from build123d import *

# Parameters (mm, degrees)
SKETCH2_R           = 1
BOSS_EXTRUDE1_DEPTH = 110


with BuildPart() as part:
    # Sketch2 → Boss-Extrude1 (new body)
    with BuildSketch(Plane.XY):
        with BuildLine():
            Line((0, 2.5), (1.335786438, 2.5))
            ThreePointArc((1.335786438, 2.5), (1.431457296, 2.519030117), (1.512563133, 2.573223305))
            Line((1.512563133, 2.573223305), (3.012563133, 4.073223305))
            ThreePointArc((3.012563133, 4.073223305), (3.066756321, 4.345670858), (2.835786438, 4.5))
            Line((2.835786438, 4.5), (1.25, 4.5))
            ThreePointArc((1.25, 4.5), (1.073223305, 4.573223305), (1, 4.75))
            Line((1, 4.75), (1, 5.75))
            ThreePointArc((1, 5.75), (1.073223305, 5.926776695), (1.25, 6))
            Line((1.25, 6), (5.75, 6))
            ThreePointArc((5.75, 6), (5.926776695, 5.926776695), (6, 5.75))
            Line((6, 5.75), (6, 1.25))
            ThreePointArc((6, 1.25), (5.926776695, 1.073223305), (5.75, 1))
            Line((5.75, 1), (4.748585621, 1))
            ThreePointArc((4.748585621, 1), (4.571808926, 1.073223305), (4.498585621, 1.25))
            Line((4.498585621, 1.25), (4.498585621, 2.834372059))
            ThreePointArc((4.498585621, 2.834372059), (4.344256479, 3.065341942), (4.071808926, 3.011148754))
            Line((4.071808926, 3.011148754), (2.573223305, 1.512563133))
            ThreePointArc((2.573223305, 1.512563133), (2.519030117, 1.431457296), (2.5, 1.335786438))
            Line((2.5, 1.335786438), (2.5, -1.335786438))
            ThreePointArc((2.5, -1.335786438), (2.519030117, -1.431457296), (2.573223305, -1.512563133))
            Line((2.573223305, -1.512563133), (4.071808926, -3.011148754))
            ThreePointArc((4.071808926, -3.011148754), (4.344256479, -3.065341942), (4.498585621, -2.834372059))
            Line((4.498585621, -2.834372059), (4.498585621, -1.25))
            ThreePointArc((4.498585621, -1.25), (4.571808926, -1.073223305), (4.748585621, -1))
            Line((4.748585621, -1), (5.75, -1))
            ThreePointArc((5.75, -1), (5.926776695, -1.073223305), (6, -1.25))
            Line((6, -1.25), (6, -5.75))
            ThreePointArc((6, -5.75), (5.926776695, -5.926776695), (5.75, -6))
            Line((5.75, -6), (1.25, -6))
            ThreePointArc((1.25, -6), (1.073223305, -5.926776695), (1, -5.75))
            Line((1, -5.75), (1, -4.75))
            ThreePointArc((1, -4.75), (1.073223305, -4.573223305), (1.25, -4.5))
            Line((1.25, -4.5), (2.835786438, -4.5))
            ThreePointArc((2.835786438, -4.5), (3.066756321, -4.345670858), (3.012563133, -4.073223305))
            Line((3.012563133, -4.073223305), (1.512563133, -2.573223305))
            ThreePointArc((1.512563133, -2.573223305), (1.431457296, -2.519030117), (1.335786438, -2.5))
            Line((1.335786438, -2.5), (-1.335786438, -2.5))
            ThreePointArc((-1.335786438, -2.5), (-1.431457296, -2.519030117), (-1.512563133, -2.573223305))
            Line((-1.512563133, -2.573223305), (-3.012563133, -4.073223305))
            ThreePointArc((-3.012563133, -4.073223305), (-3.066756321, -4.345670858), (-2.835786438, -4.5))
            Line((-2.835786438, -4.5), (-1.25, -4.5))
            ThreePointArc((-1.25, -4.5), (-1.073223305, -4.573223305), (-1, -4.75))
            Line((-1, -4.75), (-1, -5.75))
            ThreePointArc((-1, -5.75), (-1.073223305, -5.926776695), (-1.25, -6))
            Line((-1.25, -6), (-5.75, -6))
            ThreePointArc((-5.75, -6), (-5.926776695, -5.926776695), (-6, -5.75))
            Line((-6, -5.75), (-6, -1.25))
            ThreePointArc((-6, -1.25), (-5.926776695, -1.073223305), (-5.75, -1))
            Line((-5.75, -1), (-4.748585621, -1))
            ThreePointArc((-4.748585621, -1), (-4.571808926, -1.073223305), (-4.498585621, -1.25))
            Line((-4.498585621, -1.25), (-4.498585621, -2.834372059))
            ThreePointArc((-4.498585621, -2.834372059), (-4.344256479, -3.065341942), (-4.071808926, -3.011148754))
            Line((-4.071808926, -3.011148754), (-2.573223305, -1.512563133))
            ThreePointArc((-2.573223305, -1.512563133), (-2.519030117, -1.431457296), (-2.5, -1.335786438))
            Line((-2.5, -1.335786438), (-2.5, 1.335786438))
            ThreePointArc((-2.5, 1.335786438), (-2.519030117, 1.431457296), (-2.573223305, 1.512563133))
            Line((-2.573223305, 1.512563133), (-4.071808926, 3.011148754))
            ThreePointArc((-4.071808926, 3.011148754), (-4.344256479, 3.065341942), (-4.498585621, 2.834372059))
            Line((-4.498585621, 2.834372059), (-4.498585621, 1.25))
            ThreePointArc((-4.498585621, 1.25), (-4.571808926, 1.073223305), (-4.748585621, 1))
            Line((-4.748585621, 1), (-5.75, 1))
            ThreePointArc((-5.75, 1), (-5.926776695, 1.073223305), (-6, 1.25))
            Line((-6, 1.25), (-6, 5.75))
            ThreePointArc((-6, 5.75), (-5.926776695, 5.926776695), (-5.75, 6))
            Line((-5.75, 6), (-1.25, 6))
            ThreePointArc((-1.25, 6), (-1.073223305, 5.926776695), (-1, 5.75))
            Line((-1, 5.75), (-1, 4.75))
            ThreePointArc((-1, 4.75), (-1.073223305, 4.573223305), (-1.25, 4.5))
            Line((-1.25, 4.5), (-2.835786438, 4.5))
            ThreePointArc((-2.835786438, 4.5), (-3.066756321, 4.345670858), (-3.012563133, 4.073223305))
            Line((-3.012563133, 4.073223305), (-1.512563133, 2.573223305))
            ThreePointArc((-1.512563133, 2.573223305), (-1.431457296, 2.519030117), (-1.335786438, 2.5))
            Line((-1.335786438, 2.5), (0, 2.5))
        make_face()
        Circle(SKETCH2_R, mode=Mode.SUBTRACT)
    extrude(amount=-BOSS_EXTRUDE1_DEPTH)


solid = part.part
Can you work these out from the model? Positions are in its coordinate system, mm. A direction names the side the tool comes from. Coordinates: 2 decimals unless noted, no trailing zeros. Loops run counter-clockwise (first coordinate to the right, second up) from the corner with the lowest first, then second, coordinate; pieces in that order, holes last. Notation, with made-up numbers: (-16, -14.5) - (26, -14.5) arc R22 ccw to (26, 0.5) - close; hole circle Ø3 at (-39, 80). An arc over 180 degrees is marked (long way). Answer as a JSON object with one key per item and string values. Group by question number.
Item 1: If we section it at A-A (y = 0): List the corners of the cut face in (x, z) for me.
Item 2: On a 3-axis mill with a long thin cutter (end or side, diameter ignored), from which of +Z, -Z, +X, -X, +Y, -Y can I reach the whole of each face in a straight line? I mean faces 1 (the face through (0, 2.5, -54)), 2 (the face through (0.1, 1.4, 0)). Say none if no direction works.
Item 3: If we mould it in two halves opening along X, with no side actions, what happens to faces 3 (the face through (4, -6, -54)), 4 (the face through (0, -1, -54)), 5 (the face through (6, 4, -54)), 6 (the face through (0, -2.5, -54))? For each: released by +X, released by -X, zero draft, split by the parting line, or undercut.
Item 4: If I drill on L1, parallel to X at y = 1.5, z = -9; L2, parallel to Y at x = 0, z = -55; L3, parallel to Y at x = 5.25, z = -26, over which ranges is the centre line in solid material (lowest first)? Write a range as from..to.
Returned:
{
 "1": {"outline": "(-2.5, -110) - (-1, -110) - (-1, 0) - (-2.5, 0) - close; (1, -110) - (2.5, -110) - (2.5, 0) - (1, 0) - close"},
 "2": {"face 1": "+Z, -Z", "face 2": "+Z, +X, -X, +Y, -Y"},
 "3": {"face 3": "zero draft", "face 4": "undercut", "face 5": "released by +X", "face 6": "undercut"},
 "4": {"L1": "x = -6..-4.5, -2.56..2.56, 4.5..6", "L2": "y = -2.5..-1, 1..2.5", "L3": "y = -6..-1, 1..6"}
}
